Here's how the part is built. I have some questions about the finished solid (model axes, mm). Face numbers are marked on the shaded views. A direction names the side the tool comes from. Round coordinates to 2 decimals unless told otherwise and drop trailing zeros. Write each loop counter-clockwise with the first axis right and the second up, starting at its lowest first coordinate (ties: lowest second). Pieces come first, ordered by that corner, then holes. Notation, with made-up numbers: (-31.75, 41.25) -> (-26.75, 41.25) arc R22 ccw to (-26.75, 55.25) -> close; hole circle Ø9 at (45.25, -9). An arc over 180 degrees is marked (long way). Answer in a Markdown table with one row per item. Add a question column.
from build123d import *

# Parameters (mm, degrees)
SKETCH1_R           = 1.75
BOSS_EXTRUDE1_DEPTH = 5
BOSS_EXTRUDE2_START = -5
BOSS_EXTRUDE2_DEPTH = 5


with BuildPart() as part:
    # Sketch1 → Boss-Extrude1 (new body)
    with BuildSketch(Plane(origin=(0, 0, 0), x_dir=(0, 0, -1), z_dir=(1, 0, 0))):
        with BuildLine():
            Line((27, 10), (5, 10))
            ThreePointArc((5, 10), (0, 5), (5, 0))
            Line((5, 0), (27, 0))
            ThreePointArc((27, 0), (32, 5), (27, 10))
        make_face()
        with Locations((5, 5)):
            Circle(SKETCH1_R, mode=Mode.SUBTRACT)
        with Locations((27, 5)):
            Circle(SKETCH1_R, mode=Mode.SUBTRACT)
    extrude(amount=BOSS_EXTRUDE1_DEPTH)

    # Sketch2 → Boss-Extrude2 (add)
    with BuildSketch(Plane(origin=(5, 0, 0), x_dir=(0, 0, -1), z_dir=(1, 0, 0)).offset(BOSS_EXTRUDE2_START)):
        with BuildLine():
            add(Edge.make_bspline(
                [(63.752972286, 17.872423117), (45.928882678, 26.563787963), (31.059268621, 10), (13.694974759, 10)],
                knots=[0, 0, 0, 0, 1, 1, 1, 1], degree=3))
            Line((13.694974759, 10), (27, 10))
            ThreePointArc((27, 10), (31.87285141, 6.120410255), (29.183837075, 0.502127655))
            Line((29.183837075, 0.502127655), (38.08542066, 4.824084077))
            ThreePointArc((38.08542066, 4.824084077), (46.723585583, 12.05963883), (57.948000409, 11.067843667))
            Line((57.948000409, 11.067843667), (65.313809691, 14.189518476))
            Line((65.313809691, 14.189518476), (63.752972286, 17.872423117))
        make_face()
    extrude(amount=BOSS_EXTRUDE2_DEPTH)


solid = part.part
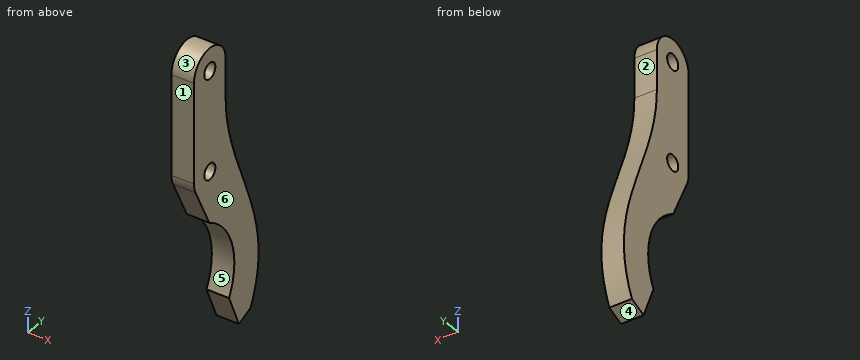
Item 1: I need wall thicknesses on line 1 along Y through (x, z) = (3.5, -5); line 2 along Z through (x, y) = (0.7, 5.5); line 3 along Y through (x, z) = (2.4, -13). Which ranges of each line are inside material? Lowest first, please. Write a range as from..to.
Item 2: On a 3-axis mill with a long thin cutter (end or side, diameter ignored), from which of +Z, -Z, +X, -X, +Y, -Y can I reach the whole of each face in a straight line? I mean the marked faces 1 and 2. Say none if no direction works.
Item 3: If we section it at A-A on x = 4.4: Give the number of separate pieces and of enclosed holes in the cut face, then the cut area to 3 significant figures.
Item 4: For P1, Ø2.5, axis at x = 1.5, z = -7, coming from the +Y side; P2, Ø3, axis at y = 5, z = -5, coming from the +X side; P3, Ø3, axis at x = 2, y = 9.5, coming from the +Z side; P4, Ø1.5, axis at x = 1, y = 3.5, coming from the +Z side, each with a flat end and sliding along its axis, tell me the tip position at first contact or that it passes through.
Item 5: If we section it at B-B on y = 2: Please give me the cut outline in (x, z).
Item 6: If we mould it in two halves opening along Z, with no side actions, what happens to the marked faces 3, 4, 5 and 6? For each: pulls with the +Z half, pulls with the -Z half, needs draft (parallel to the pull), parting line crosses it, or undercut.
Results list:
| question | item | result |
|---|---|---|
| 1 | line 1 | 0..3.25, 6.75..10 |
| 1 | line 2 | -38.46..-28.68, -25.32..-6.68, -3.32..-0.03 |
| 1 | line 3 | 0..10 |
| 2 | face 1 | +Z, -Z, +X, -X, -Y |
| 2 | face 2 | +Z, +X, -X, +Y |
| 3 | separate pieces | 1 |
| 3 | enclosed holes | 2 |
| 3 | area | 602 mm² |
| 4 | P1 | y = 10 |
| 4 | P2 | through |
| 4 | P3 | z = -1 |
| 4 | P4 | z = -0.06 |
| 5 | outline | (0, -32.27) -> (5, -32.27) -> (5, -1) -> (0, -1) -> close |
| 6 | face 3 | pulls with the +Z half |
| 6 | face 4 | pulls with the -Z half |
| 6 | face 5 | undercut |
| 6 | face 6 | needs draft |
